from build123d import *

# Parameters (mm, degrees)
BOSS_EXTRUDE1_DEPTH  = 25.4
M5_CLEARANCE_HOLE1_D = 5.5
M5_CLEARANCE_HOLE2_D = 5.5


with BuildPart() as part:
    # Sketch2 → Boss-Extrude1 (new body)
    with BuildSketch(Plane.XY):
        Polygon((0, 0), (0, 41.275), (12.7, 41.275), (12.7, 38.1), (3.175, 38.1), (3.175, 0), align=None)
    extrude(amount=BOSS_EXTRUDE1_DEPTH)

    # M5 Clearance Hole1 (through all)
    with Locations(Plane(origin=(0, 38.1, 0), x_dir=(-1, 0, 0), z_dir=(0, -1, 0))):
        with Locations((-7.9375, -12.7)):
            Hole(M5_CLEARANCE_HOLE1_D / 2)

    # M5 Clearance Hole2 (through all)
    with Locations(Plane(origin=(3.175, 0, 0), x_dir=(0, 0, -1), z_dir=(1, 0, 0))):
        with Locations((-12.7, 12.7)):
            Hole(M5_CLEARANCE_HOLE2_D / 2)


solid = part.part
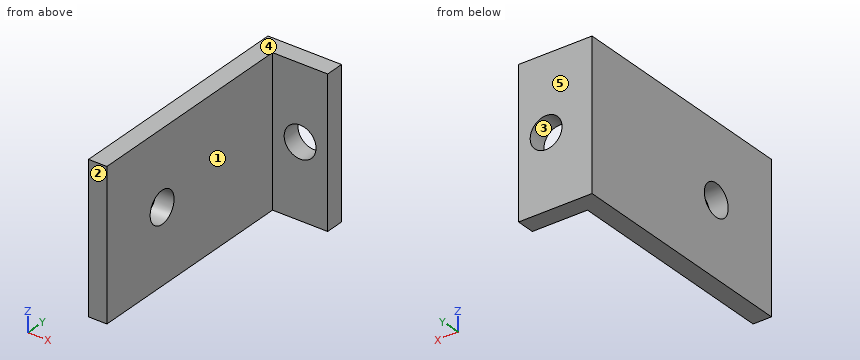
Here's how the part is built. I have some questions about the finished solid (model axes, mm). Face numbers are marked on the shaded views. A direction names the side the tool comes from. Round coordinates to 2 decimals unless told otherwise and drop trailing zeros. Write each loop counter-clockwise with the first axis right and the second up, starting at its lowest first coordinate (ties: lowest second). Pieces come first, ordered by that corner, then holes.
1. Suppose I cut it at A-A (z = 12.7). State how many separate pieces and enclosed holes the cut face has, and give its area (3 significant figures).
2. Suppose I cut it at C-C (x = 6.25). List the corners of the cut face in (y, z) for me (3 decimals), and give its area (3 significant figures).
3. Suppose I cut it at D-D (x = 2.5). List the corners of the cut face in (y, z) for me (3 decimals).
4. Will these pins go through, and if not, where does the flat tip stop? pin 1 Ø5 at (x, z) = (7.5, 7.5) entering from -Y; pin 2 Ø3.5 at (x, z) = (7.94, 12.7) entering from +Y; pin 3 Ø5 at (y, z) = (5, 17.5) entering from +X (3 decimals); pin 4 Ø9 at (y, z) = (12.7, 12.7) entering from -X.
5. If we mould it in two halves opening along Z, with no side actions, what happens to the marked faces 3, 4 and 5? For each: released by +Z, released by -Z, zero draft, split by the parting line, or undercut.
6. For the marked faces 1 and 2, which set-ups out of +Z, -Z, +X, -X, +Y, -Y let a thin tool reach every point of the face, with its end or its side?
7. I need wall thicknesses on L1, parallel to Y at x = 1.4, z = 12.7 (3 decimals); L2, parallel to X at y = 40.55, z = 12.7; L3, parallel to Y at x = 7.5, z = 9.25 (3 decimals). Which ranges of each line are inside material? Lowest first, please.
8. Suppose I cut it at B-B (y = 12.7). List the corners of the cut face in (x, z) for me (3 decimals).
Answer sheet:
1. separate pieces: 3
1. enclosed holes: 0
1. area: 126 mm2
2. outline: (38.1, 0) - (41.275, 0) - (41.275, 10.529) - (38.1, 10.529) - close; (38.1, 14.871) - (41.275, 14.871) - (41.275, 25.4) - (38.1, 25.4) - close
2. area: 66.9 mm2
3. outline: (0, 0) - (41.275, 0) - (41.275, 25.4) - (0, 25.4) - close; hole circle Ø5.5 at (12.7, 12.7)
4. pin 1: stops at y = 38.1
4. pin 2: passes through
4. pin 3: stops at x = 3.175
4. pin 4: stops at x = 0
5. face 3: undercut
5. face 4: released by +Z
5. face 5: zero draft
6. face 1: +Z, -Z, +X, -Y
6. face 2: +Z, -Z, +X, -X, -Y
7. L1: y = 0 to 9.95, 15.45 to 41.275
7. L2: x = 0 to 5.19, 10.69 to 12.7
7. L3: y = 38.1 to 41.275
8. outline: (0, 0) - (3.175, 0) - (3.175, 9.95) - (0, 9.95) - close; (0, 15.45) - (3.175, 15.45) - (3.175, 25.4) - (0, 25.4) - close
